The model under review builds one solid part; all positions refer to its coordinate system, in mm. Face numbers are marked on the shaded views. A direction names the side the tool comes from. Coordinates: 2 decimals unless noted, no trailing zeros. Write each loop counter-clockwise with the first axis right and the second up, starting at its lowest first coordinate (ties: lowest second). Pieces come first, ordered by that corner, then holes. Notation, with made-up numbers: (59, 51.5) -> (103, 51.5) arc R18 cw to (103, 70.5) -> close; hole circle Ø11 at (76.25, 15.5). An arc over 180 degrees is marked (long way). Put each result on its own line as item: value. Start each with the question number.
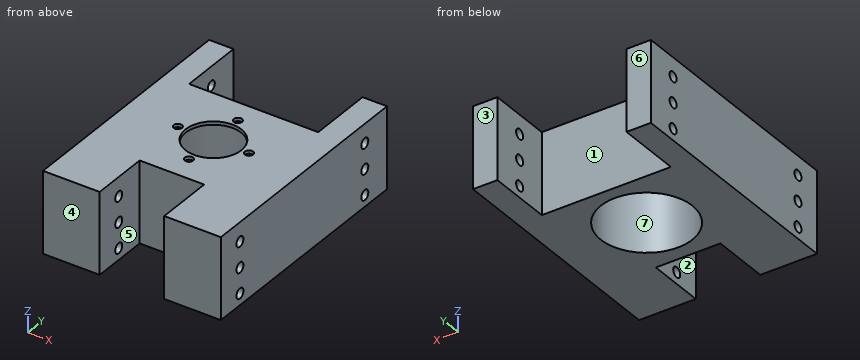
from build123d import *

# Parameters (mm, degrees)
SKETCH1_R               = 11
BOSS_EXTRUDE1_DEPTH     = 55
SKETCH2_R               = 18
CUT_EXTRUDE1_DEPTH      = 53.7
SKETCH4_R               = 1.625
CUT_EXTRUDE2_DEPTH      = 56
SKETCH5_R               = 2
CUT_EXTRUDE3_DEPTH      = 36
CUT_EXTRUDE3_DEPTH_BACK = 36
CUT_EXTRUDE4_DEPTH      = 74


with BuildPart() as part:
    # Sketch1 → Boss-Extrude1 (new body)
    with BuildSketch(Plane.XY):
        Polygon((-12.7, -23.74), (12.7, -23.74), (12.7, -46.6), (35, -46.6), (35, -20), (35, 48.4), (25.4, 48.4), (25.4, 23), (-25.4, 23), (-25.4, 48.4), (-35, 48.4), (-35, -24.5), (-35, -46.6), (-12.7, -46.6), align=None)
        Circle(SKETCH1_R, mode=Mode.SUBTRACT)
    extrude(amount=BOSS_EXTRUDE1_DEPTH)

    # Sketch2 → Cut-Extrude1 (cut)
    with BuildSketch(Plane(origin=(0, 0, 0), x_dir=(-1, 0, 0), z_dir=(0, 0, -1))):
        Circle(SKETCH2_R)
    extrude(amount=-CUT_EXTRUDE1_DEPTH, mode=Mode.SUBTRACT)

    # Sketch4 → Cut-Extrude2 (cut, through all)
    with BuildSketch(Plane.XY.offset(55)):
        with Locations((0, 14)):
            Circle(SKETCH4_R)
        with Locations((14, 0)):
            Circle(SKETCH4_R)
        with Locations((0, -14)):
            Circle(SKETCH4_R)
        with Locations((-14, 0)):
            Circle(SKETCH4_R)
    extrude(amount=-CUT_EXTRUDE2_DEPTH, mode=Mode.SUBTRACT)

    # Sketch5 → Cut-Extrude3 (cut, two sides)
    with BuildSketch(Plane(origin=(0, 0, 0), x_dir=(0, 0, -1), z_dir=(1, 0, 0))) as cut_extrude3_sk:
        with Locations((-27.5, -35.7)):
            Circle(SKETCH5_R)
        with Locations((-17.5, -35.7)):
            Circle(SKETCH5_R)
        with Locations((-7.5, -35.7)):
            Circle(SKETCH5_R)
        with Locations((-37.5, -35.7)):
            Circle(SKETCH5_R)
        with Locations((-47.5, -35.7)):
            Circle(SKETCH5_R)
        with Locations((-27.5, 35.7)):
            Circle(SKETCH5_R)
        with Locations((-37.5, 35.7)):
            Circle(SKETCH5_R)
        with Locations((-47.5, 35.7)):
            Circle(SKETCH5_R)
        with Locations((-17.5, 35.7)):
            Circle(SKETCH5_R)
        with Locations((-7.5, 35.7)):
            Circle(SKETCH5_R)
    extrude(amount=CUT_EXTRUDE3_DEPTH, mode=Mode.SUBTRACT)
    extrude(cut_extrude3_sk.sketch, amount=-CUT_EXTRUDE3_DEPTH_BACK, mode=Mode.SUBTRACT)

    # Sketch6 → Cut-Extrude4 (cut)
    with BuildSketch(Plane(origin=(35, 0, 0), x_dir=(0, 0, -1), z_dir=(1, 0, 0))):
        Polygon((-23, -1.1), (-23, 51.285793323), (26.639959918, 51.285793323), (26.639959918, -56.994126514), (-23, -56.994126514), align=None)
    extrude(amount=-CUT_EXTRUDE4_DEPTH, mode=Mode.SUBTRACT)


solid = part.part
1. Insertion check: P1, Ø6.5, axis at y = -35.7, z = 37.5, coming from the -X side; P2, Ø3, axis at y = -35.7, z = 47.5, coming from the -X side; P3, Ø3, axis at x = -4, z = 35, coming from the -Y side; P4, Ø10, axis at x = 13, z = 36.5, coming from the +Y side. Each pin has a flat end and moves straight along its axis. Give the tip position at first contact, or say it passes through.
2. Tool access review of the marked faces 1, 2 and 3: name each direction out of +Z, -Z, +X, -X, +Y, -Y from which nothing blocks a thin tool from reaching the whole face with its end or side.
3. Consider section D-D on x = 4. State the section outline as (y, z) points.
4. Consider section B-B on y = 0. State the section outline as (x, z) points (3 decimals).
5. Consider section A-A on z = 47.5. State how many separate pieces and enclosed holes the cut face has, then the cut area to 3 significant figures.
6. Wall thickness on line 1 (Z direction, x = 18, y = -35.7); line 2 (Y direction, x = 31, z = 27.5); line 3 (Z direction, x = 29, y = 35): over which ranges is each line inside the solid? List them lowest first. Write a range as from..to.
7. The part is to be moulded in two halves that separate along Y. For the marked faces 4, 5, 6 and 7, say which applies: released by +Y, released by -Y, zero draft, split by the parting line, or undercut.
8. Consider section C-C on y = -28. State the section outline as (x, z) points, then the cut area to 3 significant figures.
Output values:
1. P1: stops at x = -35
1. P2: passes through
1. P3: stops at y = -23.74
1. P4: stops at y = 23
2. face 1: +Z, -Z, +Y
2. face 2: +Z, -Z, -Y
2. face 3: +Z, -Z, +X, -X, +Y
3. outline: (-23.74, 23) -> (-17.55, 23) -> (-17.55, 53.7) -> (-10.25, 53.7) -> (-10.25, 55) -> (-23.74, 55) -> close; (10.25, 53.7) -> (17.55, 53.7) -> (17.55, 23) -> (23, 23) -> (23, 55) -> (10.25, 55) -> close
4. outline: (-35, 23) -> (-18, 23) -> (-18, 53.7) -> (-15.625, 53.7) -> (-15.625, 55) -> (-35, 55) -> close; (-12.375, 53.7) -> (-11, 53.7) -> (-11, 55) -> (-12.375, 55) -> close; (11, 53.7) -> (12.375, 53.7) -> (12.375, 55) -> (11, 55) -> close; (15.625, 53.7) -> (18, 53.7) -> (18, 23) -> (35, 23) -> (35, 55) -> (15.625, 55) -> close
5. separate pieces: 5
5. enclosed holes: 1
5. area: 3,510 mm^2
6. line 1: z = 23..25.5, 29.5..35.5, 39.5..45.5, 49.5..55
6. line 2: y = -46.6..-37.7, -33.7..33.7, 37.7..48.4
6. line 3: z = 23..25.63, 29.37..35.63, 39.37..45.63, 49.37..55
7. face 4: released by -Y
7. face 5: zero draft
7. face 6: released by +Y
7. face 7: undercut
8. outline: (-35, 23) -> (-12.7, 23) -> (-12.7, 55) -> (-35, 55) -> close; (12.7, 23) -> (35, 23) -> (35, 55) -> (12.7, 55) -> close
8. area: 1,430 mm^2
